```python
from build123d import *

# Parameters (mm, degrees)
F0_R     = 12.7
F1_DEPTH = 20.066
F2_R     = 11.43
F2_R_2   = 4.953
F3_DEPTH = 1.905
F5_D     = 2.2606
F5_DEPTH = 4.445
F5_TIP   = 0.6791527577


with BuildPart() as f1:
    # F0 (on Top) → F1 (new body)
    with BuildSketch(Plane.XY):
        Circle(F0_R)
    extrude(amount=F1_DEPTH)

    # F2 (on face) → F3 (cut)
    with BuildSketch(Plane.XY.offset(20.066)):
        Circle(F2_R)
        Circle(F2_R_2, mode=Mode.SUBTRACT)
    extrude(amount=-F3_DEPTH, mode=Mode.SUBTRACT)

    # F5
    with Locations(Plane(origin=(0, 0, 0), x_dir=(1, 0, 0), z_dir=(0, 0, -1))):
        with Locations((0, 0)):
            Hole(F5_D / 2, depth=F5_DEPTH)
            with Locations((0, 0, -(F5_DEPTH + F5_TIP / 2))):  # 118° drill point
                Cone(0, F5_D / 2, F5_TIP, mode=Mode.SUBTRACT)


solid = f1.part
```
Geometry check sheet. Reference: the model listing, model coordinates, mm. A direction names the side the tool comes from. Coordinates: 2 decimals unless noted, no trailing zeros. Write each loop counter-clockwise with the first axis right and the second up, starting at its lowest first coordinate (ties: lowest second). Pieces come first, ordered by that corner, then holes. Notation, with made-up numbers: (51, 26) -> (72, 26) arc R24 ccw to (72, 44) -> close; hole circle Ø8 at (-38, -22). An arc over 180 degrees is marked (long way). Use CSV: the item, a comma, the result in double quotes. Start each with the question number.
Item 1: Cross-section at D-D, the plane x = -2.5. Record the cut outline in (y, z), plus the area to 4 significant figures.
Item 2: Cross-section at C-C, the plane z = 10.5. Record the cut outline in (x, y), plus the area to 3 significant figures.
Item 3: Set-up check for faces 4 (the cylindrical face through (-0.64, 4.91, 19.13)), 5 (the flat face through (0, 0, 20.066)), 6 (the cylindrical face through (0.245, 1.103, 2.254)): record each of +Z, -Z, +X, -X, +Y, -Y from which the full face is reachable in a straight line by a thin tool's end or side.
Item 4: Mould release check, pull along Y, two halves, no side actions. Record for faces 1 (the flat face through (3, 0, 0)), 2 (the cylindrical face through (10.902, 3.433, 19.127)), 3 (the cylindrical face through (-2.75, -12.4, 9.89)): released by +Y, released by -Y, zero draft, split by the parting line, or undercut.
Item 5: Cross-section at B-B, the plane y = -10. Record the cut outline in (x, z), plus the area to 3 significant figures.
Item 6: Cross-section at A-A, the plane x = -5.5. Record the cut outline in (y, z), plus the area to 3 significant figures.
Item 7: Thickness scan on line 1 (Y direction, x = 0, z = 2); line 2 (Y direction, x = 0, z = 18.65); line 3 (Z direction, x = 9.75, y = 1.5). Record the ranges inside material, lowest first.
Item 8: Depth check by flat-ended pin: pin 1 Ø12 at (x, y) = (-9.5, -1) entering from +Z; pin 2 Ø6 at (x, z) = (-3.5, 4) entering from -Y; pin 3 Ø1.8 at (x, y) = (0, 0) entering from -Z; pin 4 Ø2 at (y, z) = (-9, 9.5) entering from +X. Enter the tip coordinate at first touch or a pass-through.
Answers:
1,outline,"(-12.45, 0) -> (12.45, 0) -> (12.45, 20.07) -> (11.15, 20.07) -> (11.15, 18.16) -> (4.28, 18.16) -> (4.28, 20.07) -> (-4.28, 20.07) -> (-4.28, 18.16) -> (-11.15, 18.16) -> (-11.15, 20.07) -> (-12.45, 20.07) -> close"
1,area,"473.5 mm^2"
2,outline,"circle Ø25.4 at (0, 0)"
2,area,"507 mm^2"
3,face 4,"+Z"
3,face 5,"+Z, +X, -X, +Y, -Y"
3,face 6,"-Z"
4,face 1,"zero draft"
4,face 2,"undercut"
4,face 3,"split by the parting line"
5,outline,"(-7.83, 0) -> (7.83, 0) -> (7.83, 20.07) -> (5.54, 20.07) -> (5.54, 18.16) -> (-5.54, 18.16) -> (-5.54, 20.07) -> (-7.83, 20.07) -> close"
5,area,"293 mm^2"
6,outline,"(-11.45, 0) -> (11.45, 0) -> (11.45, 20.07) -> (10.02, 20.07) -> (10.02, 18.16) -> (-10.02, 18.16) -> (-10.02, 20.07) -> (-11.45, 20.07) -> close"
6,area,"421 mm^2"
7,line 1,"-12.7 to -1.13, 1.13 to 12.7"
7,line 2,"-12.7 to -11.43, -4.95 to 4.95, 11.43 to 12.7"
7,line 3,"0 to 18.16"
8,pin 1,"z = 20.07"
8,pin 2,"y = -12.69"
8,pin 3,"z = 4.58"
8,pin 4,"x = 9.86"
